Geometry check sheet. Reference: the model listing, model coordinates, mm. Coordinates: 2 decimals unless noted, no trailing zeros. Loops run counter-clockwise (first coordinate to the right, second up) from the corner with the lowest first, then second, coordinate; pieces in that order, holes last. Notation, with made-up numbers: (77.25, -6) - (105.25, -6) arc R12 ccw to (105.25, 17) - close; hole circle Ø3 at (54, -15.5). An arc over 180 degrees is marked (long way). Write each question's results on one line, items separated by ' | '. Start each with the question number.
(1) Material ranges on probe 1 along Y at (x, z) = (-0.5, -6.5) (1 decimal); probe 2 along Z at (x, y) = (0.25, -19); probe 3 along Y at (x, z) = (-2, 44.5), recorded low to high.
(2) Sectioned sample at D-D (y = -19). Enter the section's corners in (x, z) (3 decimals).
(3) Sectioned sample at A-A (z = -51.5). Enter the section's corners in (x, y) (1 decimal), plus the area to 3 significant figures.
(4) Sectioned sample at C-C (y = 1.5). Enter the section's corners in (x, z) (1 decimal).
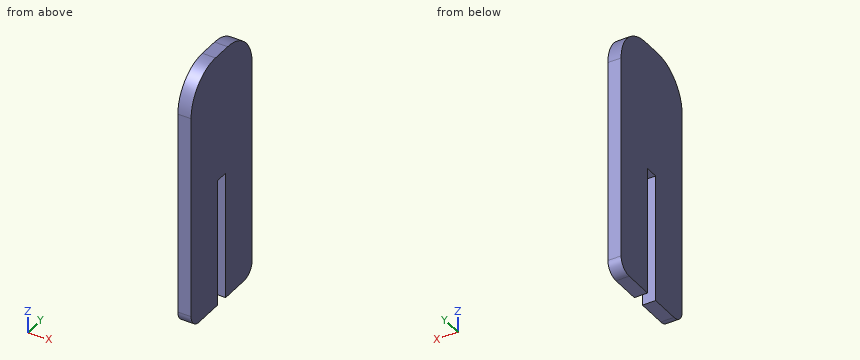
from build123d import *

# Parameters (mm, degrees)
F1_DEPTH = 3.175


with BuildPart() as f1:
    # F0 (on Right) → F1 (new body, symmetric)
    with BuildSketch(Plane.YZ):
        with BuildLine():
            Line((4.7625, 61.9125), (-4.7625, 61.9125))
            ThreePointArc((-4.7625, 61.9125), (-18.232884, 56.332884), (-23.8125, 42.8625))
            Line((-23.8125, 42.8625), (-23.8125, -55.5625))
            ThreePointArc((-23.8125, -55.5625), (-21.952628, -60.052628), (-17.4625, -61.9125))
            Line((-17.4625, -61.9125), (-3.175, -61.9125))
            Line((-3.175, -61.9125), (-3.175, 0))
            Line((-3.175, 0), (3.175, 0))
            Line((3.175, 0), (3.175, -61.9125))
            Line((3.175, -61.9125), (17.4625, -61.9125))
            ThreePointArc((17.4625, -61.9125), (21.952628, -60.052628), (23.8125, -55.5625))
            Line((23.8125, -55.5625), (23.8125, 42.8625))
            ThreePointArc((23.8125, 42.8625), (18.232884, 56.332884), (4.7625, 61.9125))
        make_face()
    extrude(amount=F1_DEPTH, both=True)


solid = f1.part
Outcome:
1) probe 1: y = -23.8 to -3.2, 3.2 to 23.8 | probe 2: z = -61.72 to 55.52 | probe 3: y = -23.74 to 23.74
2) outline: (-3.175, -61.724) - (3.175, -61.724) - (3.175, 55.519) - (-3.175, 55.519) - close
3) outline: (-3.2, -23.8) - (3.2, -23.8) - (3.2, -3.2) - (-3.2, -3.2) - close; (-3.2, 3.2) - (3.2, 3.2) - (3.2, 23.8) - (-3.2, 23.8) - close | area: 262 mm2
4) outline: (-3.2, 0) - (3.2, 0) - (3.2, 61.9) - (-3.2, 61.9) - close
